Source: CAD feature listing. Evaluate the final solid. Frame: model axes, mm. A direction names the side the tool comes from. Give positions to 0.01 mm unless a question says otherwise; leave off trailing zeros. Write each loop counter-clockwise with the first axis right and the second up, starting at its lowest first coordinate (ties: lowest second). Pieces come first, ordered by that corner, then holes. Notation, with made-up numbers: (61.25, 18) -> (87.25, 18) arc R12 cw to (87.25, 31) -> close; hole circle Ø10 at (83.25, -19.75). An arc over 180 degrees is marked (long way). Use one line per item in the form item = value. Start each with the question number.
(1) Cut plane A-A, the plane x = 32. Output: boundary loops of the cut face in (y, z).
(2) Material intervals for line 1 along Z through (x, y) = (59.7, 1.4); line 2 along X through (y, z) = (2.25, 4.5); line 3 along X through (y, z) = (-7.25, 1.5), sorted ascending. Write a range as from..to.
(3) Draft query along Z for faces 6 (the face through (60.7, 3, 4)), 7 (the face through (19.911, -1.172, 8.923)), 8 (the face through (60, -0.6, 1.2)). Return one class per face: pulls with the +Z half, pulls with the -Z half, needs draft (parallel to the pull), parting line crosses it, or undercut.
(4) Set-up query: faces 1 (the face through (61.268, -0.805, 1.006)), 2 (the face through (59.2, 1, 0)), 3 (the face through (60.35, 5.2, -6.08)), 4 (the face through (60.4, 5.4, 5.9)), 5 (the face through (-11.277, -1.799, -8.103)). Return all of +Z, -Z, +X, -X, +Y, -Y with unobstructed straight access to the full face (end or side cutting, diameter ignored); none if empty.
(5) Cut plane B-B, the plane x = 57. Output: boundary loops of the cut face in (y, z).
(6) First-contact query: P1, Ø0.9, axis at x = 60.5, y = 1, coming from the -Z side; P2, Ø0.6, axis at x = 60, y = 1, coming from the +Z side; P3, Ø6, axis at x = 50, y = 3.5, coming from the -Z side. Flat tips, straight axial feed; report the tip coordinate or a pass-through.
Autodesk Inventor part; units mm, degrees
ref_plane "ip1_XY" through (0, 0, 0) normal (1, 0, 0) x (0, 0, -1)
ref_plane "ip1_YZ" through (0, 0, 0) normal (0, 0, -1) x (0, 1, 0)
ref_plane "ip1_ZX" through (0, 0, 0) normal (0, 1, 0) x (1, 0, 0)
sketch "Sketch_1" plane through (0, 0, 0) normal (0, 0, 1) x (1, 0, 0)
  line L0 (60, 0) -> (-12.5, 0)
  line L1 (-12.5, 0) -> (-12.5, 7.8757)
  line L2 (-12.5, 7.8757) -> (-12.0757, 8.3)
  line L3 (-12.0757, 8.3) -> (-10.5, 8.3)
  line L4 (-10.5, 8.3) -> (-10.5, 8.3865)
  line L5 (-10.5, 8.3865) -> (-9.8865, 9)
  line L6 (-9.8865, 9) -> (48.8865, 9)
  line L7 (48.8865, 9) -> (49.5, 8.3865)
  line L8 (49.5, 8.3865) -> (49.5, 8.3)
  line L9 (49.5, 8.3) -> (58.97, 8.3)
  line L10 (58.97, 8.3) -> (58.97, 8.15)
  line L11 (58.97, 8.15) -> (59.5, 8.15)
  line L12 (59.5, 8.15) -> (60, 8.05)
  line L13 (60, 8.05) -> (60, 0)
  line L14 (60, 0) -> (-12.5, 0)
revolve "Revolution1" add sketch "Sketch_1" angle 360 about axis through (60, 0, 0) along (1, 0, 0)
thread "Thread1"
sketch "Sketch_2" plane through (0, 0, 0) normal (0, 0, 1) x (1, 0, 0)
  line L0 (75, -4) -> (60, -4)
  line L1 (60, -4) -> (60, -0.65)
  line L2 (60, -0.65) -> (62.5, -0.65)
  line L3 (62.5, -0.65) -> (62.5, -1.75)
  line L4 (62.5, -1.75) -> (75, -1.75)
  line L5 (75, -1.75) -> (75, -4)
  line L6 (75, -4) -> (60, -4)
revolve "Revolution2" add sketch "Sketch_2" angle 360 about axis through (75, -4, 0) along (1, 0, 0)
sketch "Sketch_5" plane through (60.7, 0, 0) normal (1, 0, 0) x (0, 0, -1)
  line L0 (1.4, 7.8765) -> (1.4, 0)
  line L1 (1.4, 0) -> (7.6942, 0)
  arc A0 (7.6942, 0) -> (7.9939, 0.3117) centre (7.6942, 0.3) ccw
  arc A1 (7.9939, 0.3117) -> (1.4, 7.8765) centre (0, 0) ccw
extrude "Extrusion1" add sketch "Sketch_5" against normal blind 0.7
sketch "Sketch_9" plane through (60.7, 0, 0) normal (1, 0, 0) x (0, 0, -1)
  arc A0 (-7.9822, 0.5333) -> (-7.4833, 0) centre (-7.4833, 0.5) ccw
  line L0 (-7.4833, 0) -> (-1.4026, 0)
  line L1 (-1.4026, 0) -> (-1.4026, 7.8761)
  arc A1 (-1.4026, 7.8761) -> (-7.9822, 0.5333) centre (0, 0) ccw
extrude "Extrusion2" add sketch "Sketch_9" against normal blind 0.7
sketch "Sketch_10" plane through (60.7, 0, 0) normal (1, 0, 0) x (0, 0, -1)
  circle A0 centre (0, 1.4) radius 1.4
extrude "Extrusion3" cut sketch "Sketch_10" against normal blind 1.5
sketch "Sketch_6" plane through (60.7, 0, 0) normal (1, 0, 0) x (0, 0, -1)
  line L0 (-0.25, 0) -> (0.25, 0)
  line L1 (0.25, 0) -> (0.25, 2.8)
  line L2 (0.25, 2.8) -> (-0.25, 2.8)
  line L3 (-0.25, 2.8) -> (-0.25, 0)
extrude "Extrusion4" add sketch "Sketch_6" against normal blind 1.1
ref_plane "ip1_XY" through (0, 0, 0) normal (1, 0, 0) x (0, 0, -1)
ref_plane "ip1_YZ" through (0, 0, 0) normal (0, 0, -1) x (0, 1, 0)
ref_plane "ip1_ZX" through (0, 0, 0) normal (0, 1, 0) x (1, 0, 0)
properties part number "BALLUFF BCS M18BBN1-PSC80D-EP021"
Geometry says:
q1.outline = circle Ø18 at (0, 0)
q2.line_1 = -7.99..-1.4, -0.25..0.25, 1.4..7.99
q2.line_2 = -12.5..60.7
q2.line_3 = -12.5..60
q3.face_6 = needs draft
q3.face_7 = parting line crosses it
q3.face_8 = undercut
q4.face_1 = +X
q4.face_2 = none
q4.face_3 = -Z, +X, +Y
q4.face_4 = +Z, +X, +Y
q4.face_5 = -X
q5.outline = circle Ø16.6 at (0, 0)
q6.P1 = -7.98
q6.P2 = 8.06
q6.P3 = -8.97
